Work out the finished part from the listing and answer in its coordinate system (mm). A direction names the side the tool comes from. Give positions to 0.01 mm unless a question says otherwise; leave off trailing zeros. Loops run counter-clockwise (first coordinate to the right, second up) from the corner with the lowest first, then second, coordinate; pieces in that order, holes last. Notation, with made-up numbers: (6, 72) - (32, 72) arc R8 cw to (32, 85) - close; hole circle Ø10 at (23, -16). An arc over 180 degrees is marked (long way). One line per question, with ' | ' between items.
from build123d import *

# Parameters (mm, degrees)
BOSS_EXTRUDE1_DEPTH     = 76.2
SKETCH3_W               = 6.35
SKETCH3_H               = 30.48
CUT_EXTRUDE1_DEPTH      = 31.75
LPATTERN11_COUNT        = 2
LPATTERN11_PITCH        = 8.255
SKETCH4_W               = 41.91
SKETCH4_H               = 33.655
BOSS_EXTRUDE2_DEPTH     = 16.51
SKETCH5_W               = 30.48
SKETCH5_H               = 6.35
CUT_EXTRUDE2_DEPTH      = 31.75
SKETCH6_R               = 1.35
CUT_EXTRUDE3_DEPTH      = 5
SKETCH9_W               = 8.255
SKETCH9_H               = 55.88
CUT_EXTRUDE5_DEPTH      = 2.5
LPATTERN12_COUNT        = 2
LPATTERN12_PITCH        = 8.255
MIRROR3_COPY_1_SKETCH_W = 6.35
MIRROR3_COPY_1_SKETCH_H = 30.48
MIRROR3_COPY_1_DEPTH    = 31.75
MIRROR3_COPY_2_SKETCH_W = 30.48
MIRROR3_COPY_2_SKETCH_H = 6.35
MIRROR3_COPY_2_DEPTH    = 31.75


with BuildPart() as part:
    # Sketch2 → Boss-Extrude1 (new body)
    with BuildSketch(Plane.XY):
        Polygon((0, 0), (41.91, 0), (41.91, 33.655), (25.4, 33.655), (25.4, 27.9), (17.145, 27.9), (17.145, 25.4), (0, 25.4), align=None)
    boss_extrude1 = extrude(amount=-BOSS_EXTRUDE1_DEPTH)

    # Sketch3 → Cut-Extrude1 (cut)
    with BuildSketch(Plane(origin=(0, 33.655, 0), x_dir=(1, 0, 0), z_dir=(0, 1, 0))):
        with Locations((29.5275, 19.05)):
            Rectangle(SKETCH3_W, SKETCH3_H)
        with Locations((29.5275, 57.15)):
            Rectangle(SKETCH3_W, SKETCH3_H)
    cut_extrude1 = extrude(amount=-CUT_EXTRUDE1_DEPTH, mode=Mode.SUBTRACT)

    # LPattern11: Cut-Extrude1 ×2
    with Locations(*[(i * LPATTERN11_PITCH, 0, 0) for i in range(1, LPATTERN11_COUNT)]):
        add(cut_extrude1, mode=Mode.SUBTRACT)

    # Sketch4 → Boss-Extrude2 (add)
    with BuildSketch(Plane(origin=(0, 0, -76.2), x_dir=(-1, 0, 0), z_dir=(0, 0, -1))):
        with Locations((-20.955, 16.8275)):
            Rectangle(SKETCH4_W, SKETCH4_H)
    boss_extrude2 = extrude(amount=BOSS_EXTRUDE2_DEPTH)

    # Sketch5 → Cut-Extrude2 (cut)
    with BuildSketch(Plane(origin=(0, 33.655, 0), x_dir=(1, 0, 0), z_dir=(0, 1, 0))):
        with Locations((16.51, 80.3275)):
            Rectangle(SKETCH5_W, SKETCH5_H)
    cut_extrude2 = extrude(amount=-CUT_EXTRUDE2_DEPTH, mode=Mode.SUBTRACT)

    # Sketch6 → Cut-Extrude3 (cut)
    with BuildSketch(Plane(origin=(0, 27.9, 0), x_dir=(1, 0, 0), z_dir=(0, 1, 0))):
        with Locations(Location((20.32, 5.08, 0), (0, 0, 270))):
            Circle(SKETCH6_R)
        with Locations(Location((20.32, 71.12, 0), (0, 0, 270))):
            Circle(SKETCH6_R)
    cut_extrude3 = extrude(amount=-CUT_EXTRUDE3_DEPTH, mode=Mode.SUBTRACT)

    # Sketch9 → Cut-Extrude5 (cut)
    with BuildSketch(Plane(origin=(0, 27.9, 0), x_dir=(1, 0, 0), z_dir=(0, 1, 0))):
        with Locations((21.2725, 38.1)):
            Rectangle(SKETCH9_W, SKETCH9_H)
    cut_extrude5 = extrude(amount=-CUT_EXTRUDE5_DEPTH, mode=Mode.SUBTRACT)

    # LPattern12: Cut-Extrude2 ×2
    with Locations(*[(0, 0, -i * LPATTERN12_PITCH) for i in range(1, LPATTERN12_COUNT)]):
        add(cut_extrude2, mode=Mode.SUBTRACT)

    # Mirror3: Boss-Extrude1, Cut-Extrude1, Boss-Extrude2, Cut-Extrude2, Cut-Extrude3, Cut-Extrude5 across plane
    add(boss_extrude1.mirror(Plane(origin=(0, 25.4, -76.2), x_dir=(0, 0, 1), z_dir=(-1, 0, 0))))
    add(cut_extrude1.mirror(Plane(origin=(0, 25.4, -76.2), x_dir=(0, 0, 1), z_dir=(-1, 0, 0))), mode=Mode.SUBTRACT)
    add(boss_extrude2.mirror(Plane(origin=(0, 25.4, -76.2), x_dir=(0, 0, 1), z_dir=(-1, 0, 0))))
    add(cut_extrude2.mirror(Plane(origin=(0, 25.4, -76.2), x_dir=(0, 0, 1), z_dir=(-1, 0, 0))), mode=Mode.SUBTRACT)
    add(cut_extrude3.mirror(Plane(origin=(0, 25.4, -76.2), x_dir=(0, 0, 1), z_dir=(-1, 0, 0))), mode=Mode.SUBTRACT)
    add(cut_extrude5.mirror(Plane(origin=(0, 25.4, -76.2), x_dir=(0, 0, 1), z_dir=(-1, 0, 0))), mode=Mode.SUBTRACT)

    # Mirror3 copy 1 sketch → Mirror3 copy 1 (cut)
    with BuildSketch(Plane(origin=(-8.255, 33.655, 0), x_dir=(-1, 0, 0), z_dir=(0, 1, 0))):
        with Locations((29.5275, -19.05)):
            Rectangle(MIRROR3_COPY_1_SKETCH_W, MIRROR3_COPY_1_SKETCH_H)
        with Locations((29.5275, -57.15)):
            Rectangle(MIRROR3_COPY_1_SKETCH_W, MIRROR3_COPY_1_SKETCH_H)
    extrude(amount=-MIRROR3_COPY_1_DEPTH, mode=Mode.SUBTRACT)

    # Mirror3 copy 2 sketch → Mirror3 copy 2 (cut)
    with BuildSketch(Plane(origin=(0, 33.655, -8.255), x_dir=(-1, 0, 0), z_dir=(0, 1, 0))):
        with Locations((16.51, -80.3275)):
            Rectangle(MIRROR3_COPY_2_SKETCH_W, MIRROR3_COPY_2_SKETCH_H)
    extrude(amount=-MIRROR3_COPY_2_DEPTH, mode=Mode.SUBTRACT)


solid = part.part
1. Which of the six approach directions +Z, -Z, +X, -X, +Y, -Y give full straight-line access (tool end or side, diameter ignored) to faces 3 (the flat face through (0, 33.655, -77)), 4 (the flat face through (-38, 18, -34.29)), 5 (the flat face through (-22, 27.9, -5))?
Evaluation:
face 3: +Z, -Z, +X, -X, +Y | face 4: +Y | face 5: +Z, +Y
2. Find section B-B on z = -55. Write down the section's boundary in (x, y) (1 decimal), then the cut area to 3 significant figures.
Evaluation:
outline: (-41.9, 0) - (41.9, 0) - (41.9, 33.7) - (41, 33.7) - (41, 1.9) - (34.6, 1.9) - (34.6, 33.7) - (32.7, 33.7) - (32.7, 1.9) - (26.4, 1.9) - (26.4, 33.7) - (25.4, 33.7) - (25.4, 25.4) - (-25.4, 25.4) - (-25.4, 33.7) - (-26.4, 33.7) - (-26.4, 1.9) - (-32.7, 1.9) - (-32.7, 33.7) - (-34.6, 33.7) - (-34.6, 1.9) - (-41, 1.9) - (-41, 33.7) - (-41.9, 33.7) - close | area: 1,600 mm2
3. Find section D-D on x = -24. Write down the section's boundary in (y, z) (1 decimal), then the cut area to 3 significant figures.
Evaluation:
outline: (0, -92.7) - (33.7, -92.7) - (33.7, -91.8) - (1.9, -91.8) - (1.9, -85.4) - (33.7, -85.4) - (33.7, -83.5) - (1.9, -83.5) - (1.9, -77.2) - (33.7, -77.2) - (33.7, -76.2) - (27.9, -76.2) - (27.9, -66) - (25.4, -66) - (25.4, -10.2) - (27.9, -10.2) - (27.9, 0) - (0, 0) - close | area: 2,140 mm2
4. Find section C-C on y = 9.5. State how many separate pieces and enclosed holes the cut face has, then the cut area to 3 significant figures.
Evaluation:
separate pieces: 1 | enclosed holes: 12 | area: 5,450 mm2
5. Determine the mould class of faces 1 (the flat face through (17.145, 27, -71)), 2 (the flat face through (31.75, 18, -80)) for opening direction Z: +Z half, -Z half, draft (parallel to the pull), parting line (faces both ways), or undercut.
Evaluation:
face 1: draft | face 2: undercut
6. Flat-ended cylindrical pins translate along their axes: pin 1 (2.5 mm diameter, centred on x = 20.32, z = -5.08, fed in from +Y); pin 2 (12 mm diameter, centred on x = 15.5, z = -11, fed in from +Y). Find the tip coordinate at first contact, or state that the pin passes through.
Evaluation:
pin 1: y = 22.9 | pin 2: y = 27.9
7. Consider L1, parallel to X at y = 2.5, z = -63; L2, parallel to X at y = 26, z = -45; L3, parallel to Z at x = -20.32, y = 26.75. Determine where each line is inside the solid, lowest interval first.
Evaluation:
L1: -41.91 to -40.96, -34.61 to -32.7, -26.35 to 26.35, 32.7 to 34.61, 40.96 to 41.91 | L2: -41.91 to -40.96, -34.61 to -32.7, -26.35 to -25.4, 25.4 to 26.35, 32.7 to 34.61, 40.96 to 41.91 | L3: -92.71 to -91.76, -85.41 to -83.5, -77.15 to -72.47, -69.77 to -66.04, -10.16 to -6.43, -3.73 to 0
8. Find section A-A on x = -12.5. Write down the section's boundary in (y, z) (1 decimal).
Evaluation:
outline: (0, -92.7) - (33.7, -92.7) - (33.7, -91.8) - (1.9, -91.8) - (1.9, -85.4) - (33.7, -85.4) - (33.7, -83.5) - (1.9, -83.5) - (1.9, -77.2) - (33.7, -77.2) - (33.7, -76.2) - (25.4, -76.2) - (25.4, 0) - (0, 0) - close
